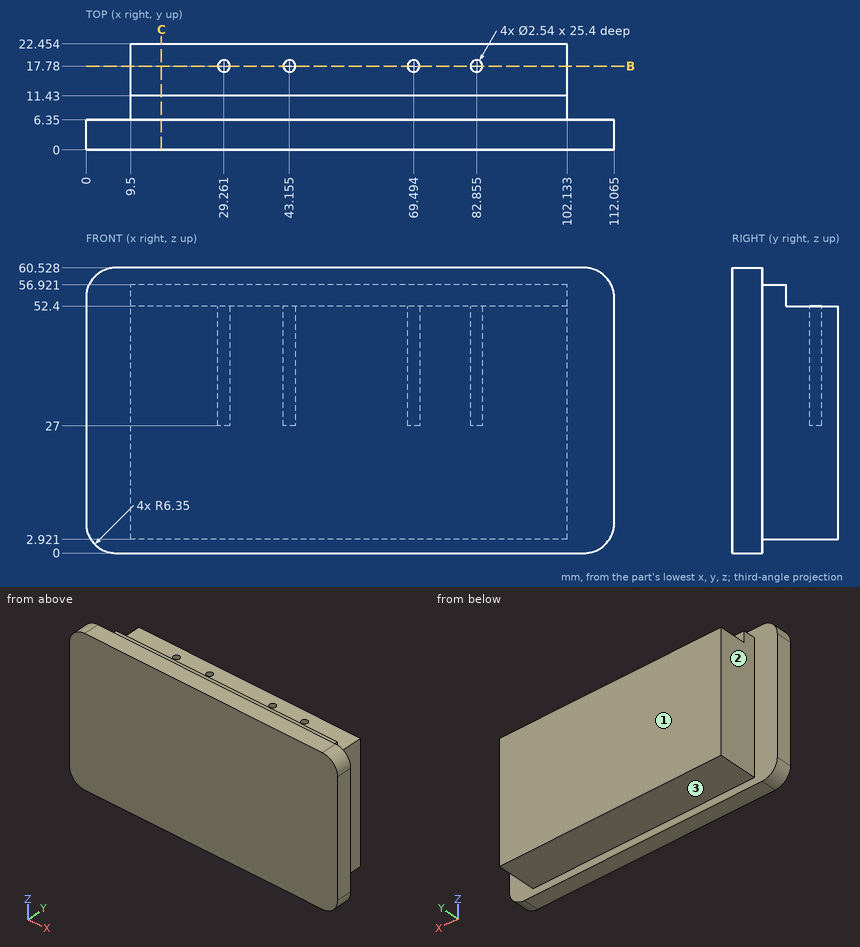
Geometry check sheet. Reference: drawing and pictorial views, mm from the part's lowest x, y, z. A direction names the side the tool comes from. Round coordinates to 2 decimals unless told otherwise and drop trailing zeros. Order: outer loops, then holes, each group sorted by start corner. A loop starts at its lowest first (then second) coordinate and runs counter-clockwise, first axis right, second up. Notation, with made-up numbers: (-32, 40) - (-4, 40) arc R30 ccw to (-4, 67) - close; hole circle Ø4 at (-22, 45.25). An arc over 180 degrees is marked (long way). One line per question, with ' | ' between items. Start each with the question number.
(1) Thickness scan on L1, parallel to Z at x = 16.5, y = 16.75; L2, parallel to X at y = 13.5, z = 32; L3, parallel to Z at x = 41, y = 9.75. Record the ranges inside material, lowest first. Write a range as [from, to].
(2) Access from +Z, -Z, +X, -X, +Y, -Y to the whole of each face (thin tool, end or side, straight path). Record for the marked faces 1, 2 and 3.
(3) Sectioned sample at B-B on y = 17.78. Record the cut outline in (x, z) (1 decimal).
(4) Sectioned sample at C-C on x = 16. Record the cut outline in (y, z), and give its area (3 significant figures).
(5) Depth check by flat-ended pin: pin 1 Ø1.3 at (x, y) = (83.5, 18) entering from +Z; pin 2 Ø3.5 at (x, z) = (61, 54) entering from +Y; pin 3 Ø8 at (y, z) = (20, 30) entering from -X; pin 4 Ø12 at (x, y) = (76.5, 14.5) entering from +Z. Enter the tip coordinate at first touch or a pass-through.
Conclusion:
1) L1: z = [2.92, 52.4] | L2: x = [9.5, 102.13] | L3: z = [2.92, 56.92]
2) face 1: +Z, -Z, +X, -X, +Y | face 2: +Z, -Z, -X, +Y | face 3: -Z, +X, -X, +Y
3) outline: (9.5, 2.9) - (102.1, 2.9) - (102.1, 52.4) - (84.1, 52.4) - (84.1, 27) - (81.6, 27) - (81.6, 52.4) - (70.8, 52.4) - (70.8, 27) - (68.2, 27) - (68.2, 52.4) - (44.4, 52.4) - (44.4, 27) - (41.9, 27) - (41.9, 52.4) - (30.5, 52.4) - (30.5, 27) - (28, 27) - (28, 52.4) - (9.5, 52.4) - close
4) outline: (0, 0) - (6.35, 0) - (6.35, 2.92) - (22.45, 2.92) - (22.45, 52.4) - (11.43, 52.4) - (11.43, 56.92) - (6.35, 56.92) - (6.35, 60.53) - (0, 60.53) - close | area: 1,200 mm2
5) pin 1: stops at z = 52.4 | pin 2: stops at y = 22.45 | pin 3: stops at x = 9.5 | pin 4: stops at z = 56.92
